from build123d import *

# Parameters (mm, degrees)
F0_W     = 127
F0_H     = 25.4
F1_DEPTH = 27.94
F2_W     = 122.428
F2_H     = 20.828
F3_DEPTH = 25.4
F4_R     = 2.54
F5_R     = 3.81


with BuildPart() as f1:
    # F0 (on Top) → F1 (new body)
    with BuildSketch(Plane.XY):
        Rectangle(F0_W, F0_H)
    extrude(amount=F1_DEPTH)

    # F2 (on face) → F3 (cut)
    with BuildSketch(Plane.XY.offset(27.94)):
        Rectangle(F2_W, F2_H)
    extrude(amount=-F3_DEPTH, mode=Mode.SUBTRACT)

    # F4
    f4_edges = [f1.edges().sort_by_distance(p)[0] for p in [
        (0, 10.414, 2.54),
        (-61.214, 0, 2.54),
        (0, -10.414, 2.54),
        (61.214, 0, 2.54),
        (-61.214, 10.414, 15.24),
        (61.214, 10.414, 15.24),
        (61.214, -10.414, 15.24),
        (-61.214, -10.414, 15.24),
    ]]
    fillet(f4_edges, radius=F4_R)

    # F5
    f5_edges = [f1.edges().sort_by_distance(p)[0] for p in [
        (-63.5, -12.7, 13.97),
        (-63.5, 12.7, 13.97),
        (63.5, 12.7, 13.97),
        (63.5, -12.7, 13.97),
    ]]
    fillet(f5_edges, radius=F5_R)


solid = f1.part
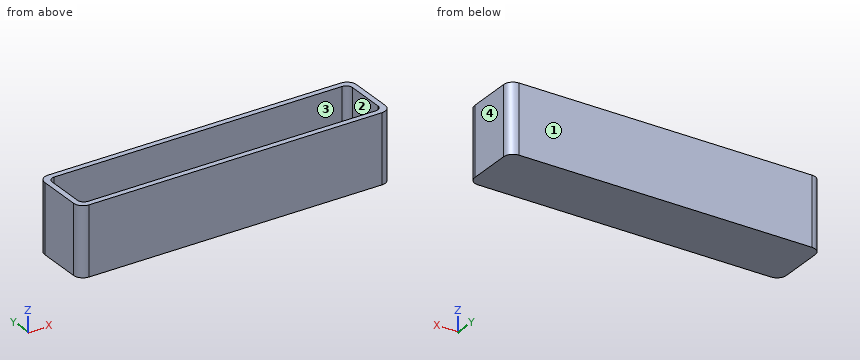
Check sheet for the modelled part. Datum: model origin and axes. Units: mm. Face numbers are marked on the shaded views. Give positions to 0.01 mm unless a question says otherwise; leave off trailing zeros. Write each loop counter-clockwise with the first axis right and the second up, starting at its lowest first coordinate (ties: lowest second). Pieces come first, ordered by that corner, then holes. Notation, with made-up numbers: (88, -40) -> (130, -40) arc R14 ccw to (130, -17) -> close; hole circle Ø8 at (-7.5, -1). An arc over 180 degrees is marked (long way). Write item = value, one per line.
Item 1: Release check for a two-part mould opening along X. For the marked faces 1, 2, 3 and 4 record: +X half, -X half, draft (parallel to the pull), parting line (faces both ways), or undercut.
Output:
face_1 = draft
face_2 = undercut
face_3 = undercut
face_4 = +X half
Item 2: Gauge pin test, flat ends, axial feed: pin 1 (5 mm diameter, centred on x = -14.5, y = -3, fed in from +Z); pin 2 (12.5 mm diameter, centred on x = -19.5, y = -3.5, fed in from +Z); pin 3 (2 mm diameter, centred on x = -30.5, y = 8.5, fed in from +Z). Record the tip position at first contact, or that the pin passes through.
Output:
pin_1 = 2.54
pin_2 = 3.37
pin_3 = 3.13
Item 3: Sectioned sample at C-C on x = -49. Record the boundary of the cut face in (y, z).
Output:
outline = (-12.7, 0) -> (12.7, 0) -> (12.7, 27.94) -> (10.41, 27.94) -> (10.41, 5.08) arc R2.54 cw to (7.87, 2.54) -> (-7.87, 2.54) arc R2.54 cw to (-10.41, 5.08) -> (-10.41, 27.94) -> (-12.7, 27.94) -> close
Item 4: Scan lines: probe 1 along X at (y, z) = (-7.25, 15); probe 2 along Y at (x, z) = (0, 16); probe 3 along X at (y, z) = (5.25, 2.75). Record each from-to range of solid material in increasing order. Write a range as from..to.
Output:
probe_1 = -63.5..-61.21, 61.21..63.5
probe_2 = -12.7..-10.41, 10.41..12.7
probe_3 = -63.5..-59.69, 59.69..63.5
Item 5: Sectioned sample at A-A on z = 24.75. Record the boundary of the cut face in (x, y), and give its area (3 significant figures).
Output:
outline = (-63.5, -8.89) arc R3.81 ccw to (-59.69, -12.7) -> (59.69, -12.7) arc R3.81 ccw to (63.5, -8.89) -> (63.5, 8.89) arc R3.81 ccw to (59.69, 12.7) -> (-59.69, 12.7) arc R3.81 ccw to (-63.5, 8.89) -> close; hole (-61.21, -7.87) arc R2.54 ccw to (-58.67, -10.41) -> (58.67, -10.41) arc R2.54 ccw to (61.21, -7.87) -> (61.21, 7.87) arc R2.54 ccw to (58.67, 10.41) -> (-58.67, 10.41) arc R2.54 ccw to (-61.21, 7.87) -> close
area = 669 mm^2
Item 6: Sectioned sample at B-B on y = 3.75. Record the boundary of the cut face in (x, z).
Output:
outline = (-63.5, 0) -> (63.5, 0) -> (63.5, 27.94) -> (61.21, 27.94) -> (61.21, 5.08) arc R2.54 cw to (58.67, 2.54) -> (-58.67, 2.54) arc R2.54 cw to (-61.21, 5.08) -> (-61.21, 27.94) -> (-63.5, 27.94) -> close
